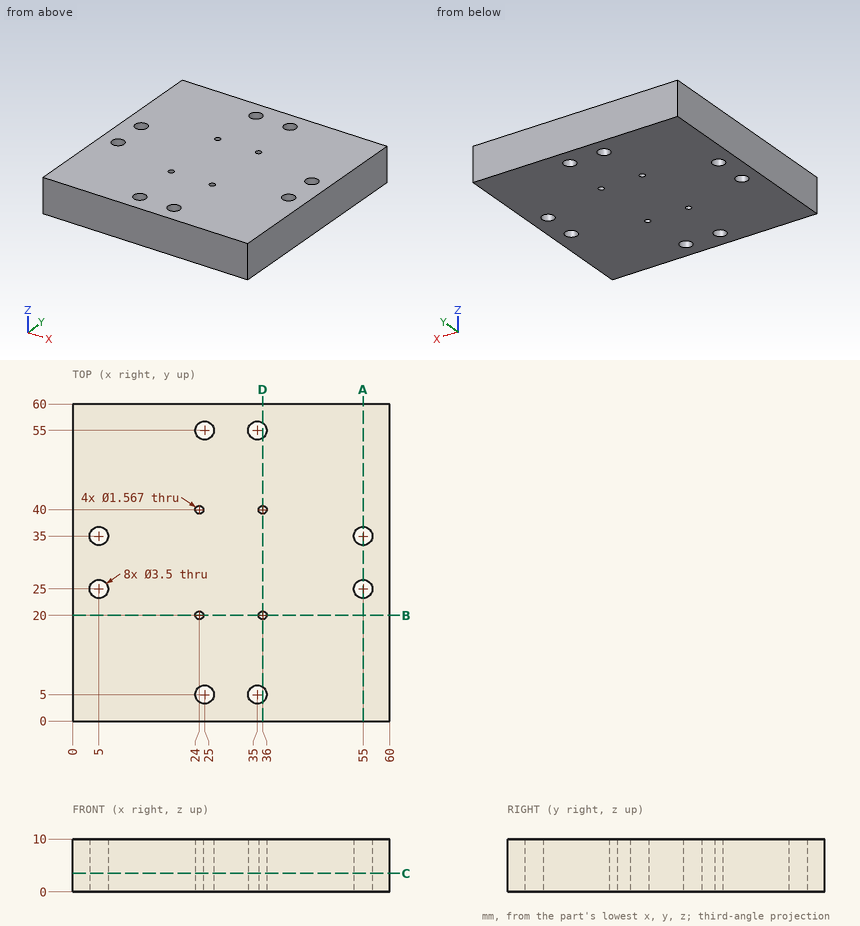
Print and shaded views of the part. All mm, measured from the part's lowest x, y and z. Coordinates: 2 decimals unless noted, no trailing zeros. Loops run counter-clockwise (first coordinate to the right, second up) from the corner with the lowest first, then second, coordinate; pieces in that order, holes last. Notation, with made-up numbers: (23.25, 60.25) -> (33.25, 60.25) arc R24 ccw to (33.25, 84.25) -> close; hole circle Ø4 at (75.5, 34.5). An arc over 180 degrees is marked (long way). Use one line per item in the form item = value. Start each with the question number.
(1) Cut at C-C on z = 3.5. Give the number of separate pieces and of enclosed holes in the cut face, and give its area (3 significant figures).
(2) Flat gauge pin, fed straight in: pin 1 (2 mm diameter, centred on x = 24, y = 40, fed in from +Z). Where does the tip first touch, or does it go through?
(3) Cut at A-A on x = 55. Give the cut face in (y, z).
(4) Probe probe 1 along X at (y, z) = (55, 7); probe 2 along X at (y, z) = (40, 5); probe 3 along Y at (x, z) = (56, 3.25). List the from-to ranges inside material, lowest first. Write a range as from..to.
(5) Cut at B-B on y = 20. Give the cut face in (x, z).
(6) Cut at D-D on x = 36. Give the cut face in (y, z), and give its area (3 significant figures).
Values:
q1.separate_pieces = 1
q1.enclosed_holes = 12
q1.area = 3,520 mm2
q2.pin_1 = 10
q3.outline = (0, 0) -> (23.25, 0) -> (23.25, 10) -> (0, 10) -> close; (26.75, 0) -> (33.25, 0) -> (33.25, 10) -> (26.75, 10) -> close; (36.75, 0) -> (60, 0) -> (60, 10) -> (36.75, 10) -> close
q4.probe_1 = 0..23.25, 26.75..33.25, 36.75..60
q4.probe_2 = 0..23.22, 24.78..35.22, 36.78..60
q4.probe_3 = 0..23.56, 26.44..33.56, 36.44..60
q5.outline = (0, 0) -> (23.22, 0) -> (23.22, 10) -> (0, 10) -> close; (24.78, 0) -> (35.22, 0) -> (35.22, 10) -> (24.78, 10) -> close; (36.78, 0) -> (60, 0) -> (60, 10) -> (36.78, 10) -> close
q6.outline = (0, 0) -> (3.56, 0) -> (3.56, 10) -> (0, 10) -> close; (6.44, 0) -> (19.22, 0) -> (19.22, 10) -> (6.44, 10) -> close; (20.78, 0) -> (39.22, 0) -> (39.22, 10) -> (20.78, 10) -> close; (40.78, 0) -> (53.56, 0) -> (53.56, 10) -> (40.78, 10) -> close; (56.44, 0) -> (60, 0) -> (60, 10) -> (56.44, 10) -> close
q6.area = 511 mm2
